from build123d import *

# Parameters (mm, degrees)
FORMED_WEB_DEPTH           = 10
EDGE_STIFFENING_LIPS_DEPTH = 206.123068282
WALL_MOUNT_HOLE_SKETCH_R   = 1.7
WALL_MOUNT_HOLES_DEPTH     = 2.4
COVER_MOUNT_HOLE_SKETCH_R  = 1.7
COVER_MOUNT_HOLE_DEPTH     = 2.4
FRAME_MOUNT_RELIEF_DEPTH   = 2.4


with BuildPart() as part:
    # Formed Web Section Sketch → Formed Web (new body)
    with BuildSketch(Plane(origin=(-30, 0, 0), x_dir=(0, 0, -1), z_dir=(1, 0, 0))):
        with BuildLine():
            Line((-22, 64), (-77.377483747, 64))
            ThreePointArc((-77.377483747, 64), (-80.010089753, 64.988457933), (-81.341585612, 67.46530719))
            Line((-81.341585612, 67.46530719), (-109.964101865, 279.66672079))
            ThreePointArc((-109.964101865, 279.66672079), (-109.991015376, 279.933465342), (-110, 280.2014136))
            Line((-110, 280.2014136), (-110, 290))
            Line((-110, 290), (-108, 290))
            Line((-108, 290), (-108, 280.2014136))
            ThreePointArc((-108, 280.2014136), (-107.995507688, 280.067439471), (-107.982050933, 279.934067195))
            Line((-107.982050933, 279.934067195), (-79.35953468, 67.732653595))
            ThreePointArc((-79.35953468, 67.732653595), (-78.69378675, 66.494228967), (-77.377483747, 66))
            Line((-77.377483747, 66), (-22, 66))
            Line((-22, 66), (-22, 64))
        make_face()
    extrude(amount=FORMED_WEB_DEPTH)

    # Edge Lip Sketch → Edge Stiffening Lips (add)
    with BuildSketch(Plane(origin=(0, 80.999511953, 10.925515566), x_dir=(-1, 0, 0), z_dir=(0, -0.9910254663478989, -0.1336732024376229))):
        with BuildLine():
            Line((34, -67.593279149), (34, -61.593279149))
            Line((34, -61.593279149), (32, -61.593279149))
            Line((32, -61.593279149), (32, -67.593279149))
            ThreePointArc((32, -67.593279149), (31.414213562, -69.007492712), (30, -69.593279149))
            Line((30, -69.593279149), (29.9, -69.593279149))
            Line((29.9, -69.593279149), (29.9, -71.593279149))
            Line((29.9, -71.593279149), (30, -71.593279149))
            ThreePointArc((30, -71.593279149), (32.828427125, -70.421706274), (34, -67.593279149))
        make_face()
        with BuildLine():
            Line((16, -67.593279149), (16, -61.593279149))
            Line((16, -61.593279149), (18, -61.593279149))
            Line((18, -61.593279149), (18, -67.593279149))
            ThreePointArc((18, -67.593279149), (18.585786438, -69.007492712), (20, -69.593279149))
            Line((20, -69.593279149), (20.1, -69.593279149))
            Line((20.1, -69.593279149), (20.1, -71.593279149))
            Line((20.1, -71.593279149), (20, -71.593279149))
            ThreePointArc((20, -71.593279149), (17.171572875, -70.421706274), (16, -67.593279149))
        make_face()
    extrude(amount=-EDGE_STIFFENING_LIPS_DEPTH)

    # Wall Mount Hole Sketch → Wall Mount Holes (cut)
    with BuildSketch(Plane(origin=(0, 63.8, 0), x_dir=(-1, 0, 0), z_dir=(0, -1, 0))):
        with Locations(Location((25, -29, 0), (0, 0, 90))):
            Circle(WALL_MOUNT_HOLE_SKETCH_R)
        with Locations(Location((25, -36, 0), (0, 0, 90))):
            Circle(WALL_MOUNT_HOLE_SKETCH_R)
    extrude(amount=-WALL_MOUNT_HOLES_DEPTH, mode=Mode.SUBTRACT)

    # Cover Mount Hole Sketch → Cover Mount Hole (cut)
    with BuildSketch(Plane.XY.offset(107.8)):
        with Locations(Location((-25, 285, 0), (0, 0, 90))):
            Circle(COVER_MOUNT_HOLE_SKETCH_R)
    extrude(amount=COVER_MOUNT_HOLE_DEPTH, mode=Mode.SUBTRACT)

    # Frame Mount Relief Sketch → Frame Mount Relief (cut)
    with BuildSketch(Plane(origin=(0, 63.8, 0), x_dir=(-1, 0, 0), z_dir=(0, -1, 0))):
        with BuildLine():
            Line((30, -36), (29.7, -36))
            ThreePointArc((29.7, -36), (28.992893219, -36.292893219), (28.7, -37))
            Line((28.7, -37), (28.7, -44))
            ThreePointArc((28.7, -44), (28.992893219, -44.707106781), (29.7, -45))
            Line((29.7, -45), (30, -45))
            ThreePointArc((30, -45), (30.707106781, -44.707106781), (31, -44))
            Line((31, -44), (31, -37))
            ThreePointArc((31, -37), (30.707106781, -36.292893219), (30, -36))
        make_face()
    extrude(amount=-FRAME_MOUNT_RELIEF_DEPTH, mode=Mode.SUBTRACT)


solid = part.part
Can you work these out from the model? Positions are in its coordinate system, mm. A direction names the side the tool comes from. Coordinates: 2 decimals unless noted, no trailing zeros. Write each loop counter-clockwise with the first axis right and the second up, starting at its lowest first coordinate (ties: lowest second). Pieces come first, ordered by that corner, then holes. Notation, with made-up numbers: (71.25, 32) - (109.25, 32) arc R21 cw to (109.25, 60) - close; hole circle Ø3 at (-21, -4). An arc over 180 degrees is marked (long way). Return JSON: item names as keys, results as strings. Group by question number.
Item 1: We'd pull the mould along X, two halves only. Please class faces 1 (the face through (-17.203, 172.289, 94.33)), 2 (the face through (-31.43, 172.48, 92.88)), 3 (the face through (-24.93, 172.081, 95.452)), 4 (the face through (-32.797, 172.289, 94.33)): pulls with the +X half, pulls with the -X half, needs draft (parallel to the pull), parting line crosses it, or undercut.
Item 2: Please list where these lines run through material, in increasing order: probe 1 along X at (y, z) = (65.1, 29); probe 2 along X at (y, z) = (112, 78); probe 3 along Y at (x, z) = (-24.75, 63.5).
Item 3: Which directions (+Z, -Z, +X, -X, +Y, -Y) give clear straight access to the entire face, cutting with the end or side of a thin tool? Please do faces 5 (the face through (-32, 173, 88)), 6 (the face through (-32.4, 72.1, 76.9)), 7 (the face through (-17.6, 72.1, 76.9)).
Item 4: If we section it at A-A (z = 58.5): Write out the boundary of the cut face in (x, y).
Item 5: I'm going to push flat-ended pins straight in: pin 1 Ø3 at (y, z) = (280.5, 109) entering from -X; pin 2 Ø2 at (x, y) = (-30, 227.5) entering from +Z; pin 3 Ø0.8 at (y, z) = (284, 109.5) entering from +X. Where does each tip first touch, or does it pass through?
Return value:
{
 "1": {"face 1": "pulls with the +X half", "face 2": "undercut", "face 3": "needs draft", "face 4": "pulls with the -X half"},
 "2": {"probe 1": "x = -30 to -26.7, -23.3 to -20", "probe 2": "x = -34 to -32, -18 to -16", "probe 3": "y = 64 to 66"},
 "3": {"face 5": "-Z, +Y", "face 6": "-Z, -X, -Y", "face 7": "-Z, +X, -Y"},
 "4": {"outline": "(-30, 64) - (-20, 64) - (-20, 66) - (-30, 66) - close"},
 "5": {"pin 1": "stops at x = -30", "pin 2": "stops at z = 103.06", "pin 3": "stops at x = -20"}
}
